Read the model definition and answer for the solid it produces. Units are mm, in the model's axes. Face numbers are marked on the shaded views. A direction names the side the tool comes from. Coordinates: 2 decimals unless noted, no trailing zeros. Loops run counter-clockwise (first coordinate to the right, second up) from the corner with the lowest first, then second, coordinate; pieces in that order, holes last. Notation, with made-up numbers: (-16.75, -21.5) -> (14.25, -21.5) arc R26 ccw to (14.25, 1.5) -> close; hole circle Ø9 at (-20, -19.5). An arc over 180 degrees is marked (long way). Answer as CSV lines item,"result".
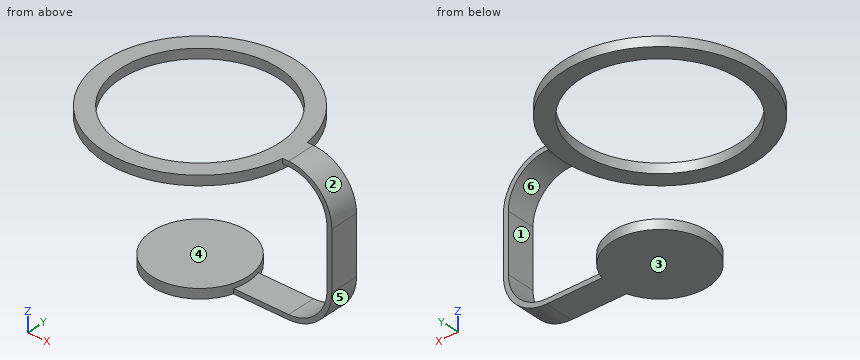
```python
from build123d import *

# Parameters (mm, degrees)
SKETCH7_R                = 10
SKETCH7_R_2              = 8.25
BOSS_EXTRUDE3_DEPTH      = 1
SKETCH8_R                = 5
BOSS_EXTRUDE4_DEPTH      = 1
BOSS_EXTRUDE5_DEPTH      = 1.5
BOSS_EXTRUDE5_DEPTH_BACK = 1.5


with BuildPart() as part:
    # Sketch7 → Boss-Extrude3 (new body)
    with BuildSketch(Plane.XY.offset(13)):
        Circle(SKETCH7_R)
        Circle(SKETCH7_R_2, mode=Mode.SUBTRACT)
    extrude(amount=BOSS_EXTRUDE3_DEPTH)



with BuildPart() as body_2:
    # Sketch8 → Boss-Extrude4 (new body)
    with BuildSketch(Plane.XY):
        Circle(SKETCH8_R)
    extrude(amount=-BOSS_EXTRUDE4_DEPTH)


with BuildPart() as part_1:
    add(part.part)

    add(body_2.part)  # Boss-Extrude5 merges body 2
    # Sketch9 → Boss-Extrude5 (add, two sides: drawn at the far end of the back side and taken through both)
    with BuildSketch(Plane(origin=(0, 0, 0), x_dir=(1, 0, 0), z_dir=(0, 1, 0)).offset(-BOSS_EXTRUDE5_DEPTH_BACK)):
        with BuildLine():
            Line((10, -13.5), (10.5, -13.5))
            ThreePointArc((10.5, -13.5), (13.328427125, -12.328427125), (14.5, -9.5))
            Line((14.5, -9.5), (14.5, -3.5))
            ThreePointArc((14.5, -3.5), (13.328427125, -0.671572875), (10.5, 0.5))
            Line((10.5, 0.5), (5, 0.5))
            Line((5, 0.5), (4.7, 0.5))
            Line((4.7, 0.5), (4.7, 1))
            Line((4.7, 1), (5, 1))
            Line((5, 1), (10.5, 1))
            ThreePointArc((10.5, 1), (13.681980515, -0.318019485), (15, -3.5))
            Line((15, -3.5), (15, -9.5))
            ThreePointArc((15, -9.5), (13.681980515, -12.681980515), (10.5, -14))
            Line((10.5, -14), (10, -14))
            Line((10, -14), (9.7, -14))
            Line((9.7, -14), (9.7, -13.5))
            Line((9.7, -13.5), (10, -13.5))
        make_face()
    extrude(amount=BOSS_EXTRUDE5_DEPTH + BOSS_EXTRUDE5_DEPTH_BACK)


solid = part_1.part
```
Q1. A cutting plane is placed at B-B, the plane x = 0. Write down the section's boundary in (y, z).
Results:
outline,"(-10, 13) -> (-8.25, 13) -> (-8.25, 14) -> (-10, 14) -> close; (-5, -1) -> (5, -1) -> (5, 0) -> (-5, 0) -> close; (8.25, 13) -> (10, 13) -> (10, 14) -> (8.25, 14) -> close"
Q2. For the marked faces 4, 5 and 6, determine the directions among +Z, -Z, +X, -X, +Y, -Y from which every point of the face is accessible in a straight line to the end or side of a thin tool.
Results:
face 4,"+Z, -X, +Y, -Y"
face 5,"-Z, +X, +Y, -Y"
face 6,"+Y, -Y"
Q3. A cutting plane is placed at D-D, the plane x = -6.5. Write down the section's boundary in (y, z), and give its area (3 significant figures).
Results:
outline,"(-7.6, 13) -> (-5.08, 13) -> (-5.08, 14) -> (-7.6, 14) -> close; (5.08, 13) -> (7.6, 13) -> (7.6, 14) -> (5.08, 14) -> close"
area,"5.04 mm²"
Q4. Given pin 1 Ø5 at (x, y) = (1.5, 1) entering from +Z; pin 2 Ø3.5 at (y, z) = (-0.5, 5.5) entering from -X; pin 3 Ø1.5 at (x, y) = (-1.5, 7.5) entering from -Z; pin 4 Ø5 at (x, z) = (-6.5, 2.5) entering from -Y, each flat-ended and moving along its own axis, determine where each tip first touches the part or whether it passes through.
Results:
pin 1,"stops at z = 0"
pin 2,"stops at x = 14.5"
pin 3,"stops at z = 13"
pin 4,"passes through"
Q5. For a pull along Z with two mould halves and no side action, classify the marked faces 1, 2 and 3 as pulls with the +Z half, pulls with the -Z half, needs draft (parallel to the pull), parting line crosses it, or undercut.
Results:
face 1,"undercut"
face 2,"pulls with the +Z half"
face 3,"pulls with the -Z half"
Q6. A cutting plane is placed at A-A, the plane y = 0. Write down the section's boundary in (x, z), and give its area (3 significant figures).
Results:
outline,"(-10, 13) -> (-8.25, 13) -> (-8.25, 14) -> (-10, 14) -> close; (-5, -1) -> (10.5, -1) arc R4.5 ccw to (15, 3.5) -> (15, 9.5) arc R4.5 ccw to (10.5, 14) -> (8.25, 14) -> (8.25, 13) -> (10, 13) -> (10, 13.5) -> (10.5, 13.5) arc R4 cw to (14.5, 9.5) -> (14.5, 3.5) arc R4 cw to (10.5, -0.5) -> (5, -0.5) -> (5, 0) -> (-5, 0) -> close"
area,"26.2 mm²"
Q7. A cutting plane is placed at C-C, the plane y = 3.25. Write down the section's boundary in (x, z), and give its area (3 significant figures).
Results:
outline,"(-9.46, 13) -> (-7.58, 13) -> (-7.58, 14) -> (-9.46, 14) -> close; (-3.8, -1) -> (3.8, -1) -> (3.8, 0) -> (-3.8, 0) -> close; (7.58, 13) -> (9.46, 13) -> (9.46, 14) -> (7.58, 14) -> close"
area,"11.3 mm²"
Q8. Find the intervals of material crossed by probe 1 along Y at (x, z) = (0, 13.85); probe 2 along X at (y, z) = (1, 9.5); probe 3 along Z at (x, y) = (14, 1), in increasing order. Write a range as [from, to].
Results:
probe 1,"y = [-10, -8.25], [8.25, 10]"
probe 2,"x = [14.5, 15]"
probe 3,"z = [0.67, 1.56], [11.44, 12.33]"
